For this review, use the dimensioned drawing (mm, ordinates from the lowest corner) and the shaded views. A direction names the side the tool comes from. Round coordinates to 2 decimals unless told otherwise and drop trailing zeros. Loops run counter-clockwise (first coordinate to the right, second up) from the corner with the lowest first, then second, coordinate; pieces in that order, holes last. Notation, with made-up numbers: (48, 88.25) -> (102, 88.25) arc R30 cw to (102, 110.25) -> close; hole circle Ø9 at (13, 63). An arc over 180 degrees is marked (long way). Answer as CSV lines item,"result". Start each with the question number.
(1) Take a section at A-A, the plane z = 89. Write out the cut boundary in (x, y) (1 decimal).
(2) Take a section at C-C, the plane x = 37. Write out the cut boundary in (y, z) (1 decimal), and give its area (3 significant figures).
(3) Machinability: for the marked faces 1, 2 and 3, which of the approach directions +Z, -Z, +X, -X, +Y, -Y give a long, thin tool a straight path to every point of the face, cutting with its end or side? Answer none if there is none.
(4) For P1, Ø3, axis at x = 16.5, z = 20.5, coming from the -Y side; P2, Ø1, axis at x = 10.5, z = 10, coming from the +Y side; P3, Ø10, axis at y = 29, z = 82, coming from the +X side, all flat-tipped, find the tip position at first contact; note any pin that passes through.
(5) To check wall thickness, follow line 1 (X direction, y = 58, z = 39); line 2 (X direction, y = 101, z = 24.5); line 3 (Y direction, x = 17.5, z = 51) (1 decimal). State the ranges of each line that lie inside material, in increasing order. Write a range as from..to.
(6) Take a section at B-B, the plane y = 66. Write out the cut boundary in (x, z), and give its area (3 significant figures).
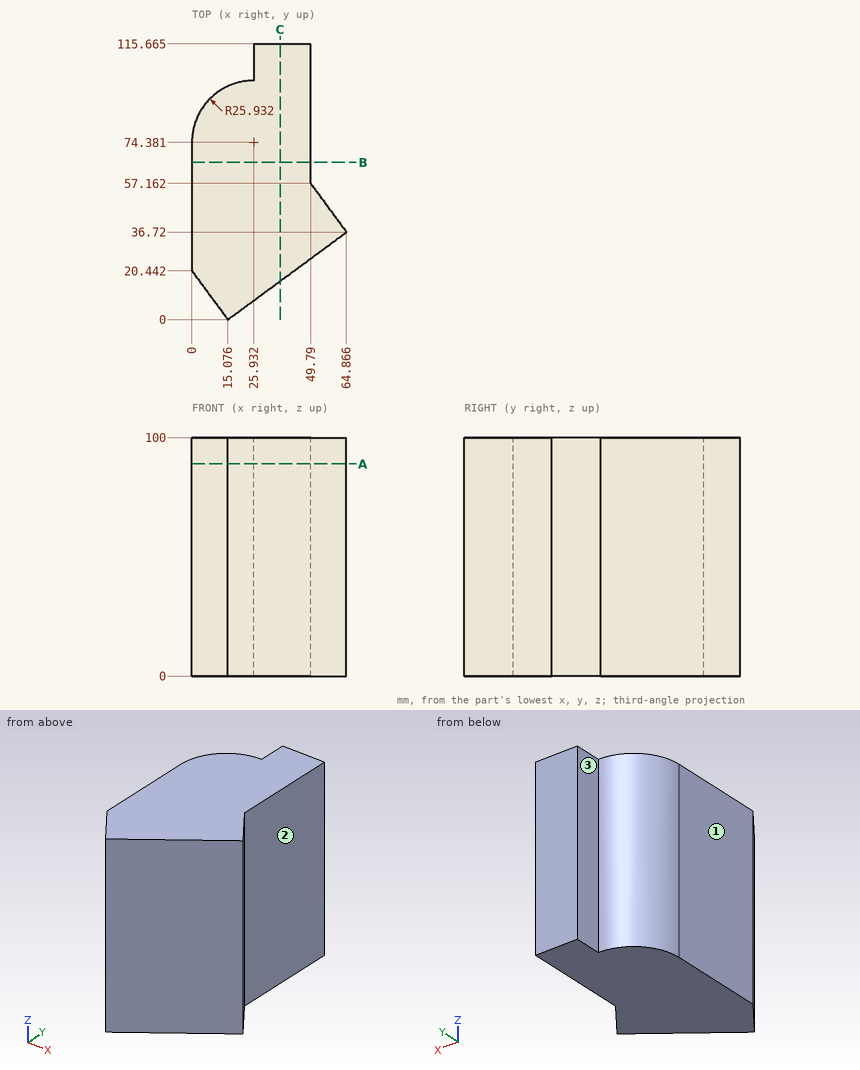
The answers:
1,outline,"(0, 20.4) -> (15.1, 0) -> (64.9, 36.7) -> (49.8, 57.2) -> (49.8, 115.7) -> (25.9, 115.7) -> (25.9, 100.3) arc R25.9 ccw to (0, 74.4) -> close"
2,outline,"(16.2, 0) -> (115.7, 0) -> (115.7, 100) -> (16.2, 100) -> close"
2,area,"9,950 mm²"
3,face 1,"+Z, -Z, -X, +Y, -Y"
3,face 2,"+Z, -Z, +X, +Y"
3,face 3,"+Z, -Z, -X, +Y"
4,P1,"y = 0"
4,P2,"y = 95.58"
4,P3,"x = 61.18"
5,line 1,"0..49.79"
5,line 2,"25.93..49.79"
5,line 3,"1.8..98.9"
6,outline,"(0, 0) -> (49.79, 0) -> (49.79, 100) -> (0, 100) -> close"
6,area,"4,980 mm²"
